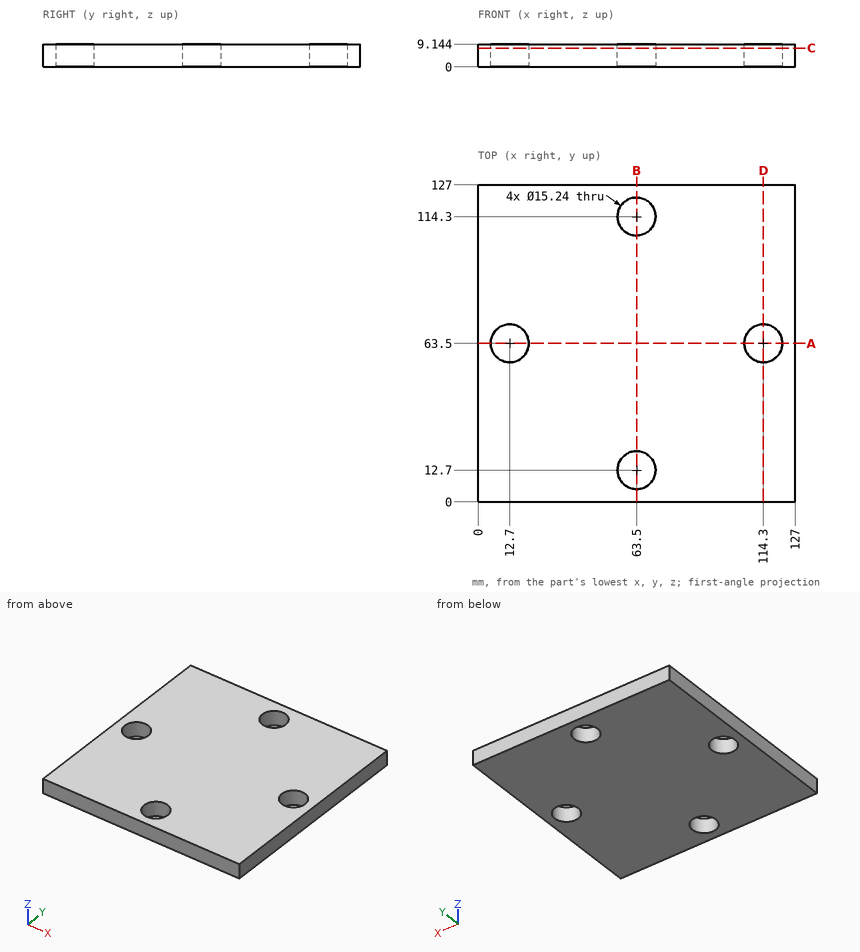
Geometry: see drawing. Coordinates: mm, zero at the bounding-box minimum. Round coordinates to 2 decimals unless told otherwise and drop trailing zeros. Write each loop counter-clockwise with the first axis right and the second up, starting at its lowest first coordinate (ties: lowest second). Pieces come first, ordered by that corner, then holes.
1) Cut plane C-C (z = 7.5). Return the cut outline in (x, y), then the cut area to 3 significant figures.
2) Cut plane A-A (y = 63.5). Return the cut outline in (x, z).
3) Ray query, L1, parallel to Y at x = 63.5, z = 4; L2, parallel to Y at x = 114.3, z = 5; L3, parallel to X at y = 6, z = 8.75. Return the intervals inside material, ascending.
4) Cut plane D-D (x = 114.3). Return the cut outline in (y, z).
Geometry says:
1. outline: (0, 0) - (127, 0) - (127, 127) - (0, 127) - close; hole circle Ø15.24 at (12.7, 63.5); hole circle Ø15.24 at (63.5, 12.7); hole circle Ø15.24 at (63.5, 114.3); hole circle Ø15.24 at (114.3, 63.5)
1. area: 15,400 mm2
2. outline: (0, 0) - (5.08, 0) - (5.08, 9.14) - (0, 9.14) - close; (20.32, 0) - (106.68, 0) - (106.68, 9.14) - (20.32, 9.14) - close; (121.92, 0) - (127, 0) - (127, 9.14) - (121.92, 9.14) - close
3. L1: y = 0 to 5.08, 20.32 to 106.68, 121.92 to 127
3. L2: y = 0 to 55.88, 71.12 to 127
3. L3: x = 0 to 59.87, 67.13 to 127
4. outline: (0, 0) - (55.88, 0) - (55.88, 9.14) - (0, 9.14) - close; (71.12, 0) - (127, 0) - (127, 9.14) - (71.12, 9.14) - close
